CAD build for the part. Positions are in the model's coordinates, mm. Face numbers are marked on the shaded views. A direction names the side the tool comes from. Round coordinates to 2 decimals unless told otherwise and drop trailing zeros. Order: outer loops, then holes, each group sorted by start corner. A loop starts at its lowest first (then second) coordinate and runs counter-clockwise, first axis right, second up. Notation, with made-up numbers: (26.25, -34) -> (71.25, -34) arc R30 cw to (71.25, 0) -> close; hole circle Ø9 at (10, 72.5). An arc over 180 degrees is marked (long way). Answer as CSV lines item,"result". Start each with the question number.
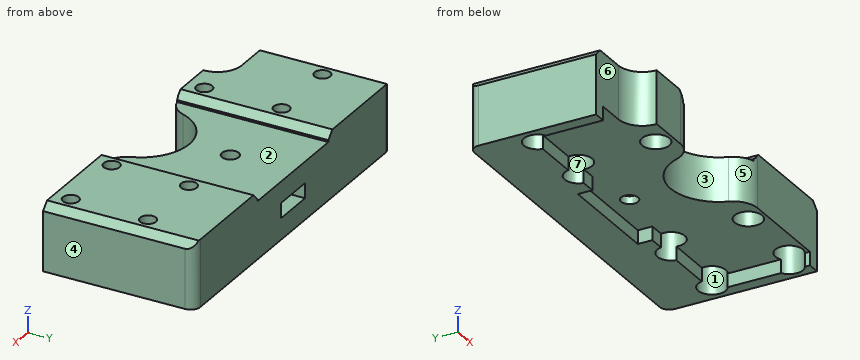
from build123d import *

# Parameters (mm, degrees)
CROQUIS1_W                  = 72
CROQUIS1_H                  = 35.8
SALIENTE_EXTRUIR1_DEPTH     = 23
CORTAR_EXTRUIR2_DEPTH       = 2.8
CROQUIS3_W                  = 5.9
CROQUIS3_H                  = 3.1
CORTAR_EXTRUIR3_DEPTH       = 7.91
SALIENTE_EXTRUIR3_DEPTH     = 3.1
CROQUIS7_W                  = 72
CROQUIS7_H                  = 22
CORTAR_EXTRUIR6_DEPTH       = 37.91
CORTAR_EXTRUIR8_DEPTH       = 15
CORTAR_EXTRUIR8_DEPTH_BACK  = 15
CROQUIS9_R                  = 1.75
CROQUIS11_R                 = 10
CORTAR_EXTRUIR10_DEPTH      = 10
REDONDEO1_R                 = 5
CROQUIS12_W                 = 72
CROQUIS12_H                 = 13.8
CROQUIS12_W_2               = 5.9
CROQUIS12_H_2               = 3.1
SALIENTE_EXTRUIR4_DEPTH     = 3.5
CROQUIS13_R                 = 1.65
CORTAR_EXTRUIR11_DEPTH      = 33.5
CORTAR_EXTRUIR12_DEPTH      = 33.5
CORTAR_EXTRUIR12_DEPTH_BACK = 3
CROQUIS14_R                 = 2.85
CROQUIS15_W                 = 26
CROQUIS15_H                 = 1.9
CORTAR_EXTRUIR13_DEPTH      = 43
CHAFL_N1_SIZE               = 1.5
CHAFL_N2_SIZE               = 1.5
CROQUIS16_W                 = 13.15
CROQUIS16_H                 = 5.14
CORTAR_EXTRUIR14_DEPTH      = 20
REDONDEO3_R                 = 5
CROQUIS17_W                 = 8.9
CROQUIS17_H                 = 3.1
SALIENTE_EXTRUIR5_DEPTH     = 4.95
REDONDEO4_R                 = 2


with BuildPart() as part:
    # Croquis1 → Saliente-Extruir1 (new body)
    with BuildSketch(Plane(origin=(0, 0, 0), x_dir=(1, 0, 0), z_dir=(0, 1, 0))):
        with Locations((36, 17.9)):
            Rectangle(CROQUIS1_W, CROQUIS1_H)
    extrude(amount=SALIENTE_EXTRUIR1_DEPTH)

    # Croquis2 → Cortar-Extruir2 (cut)
    with BuildSketch(Plane(origin=(0, 0, -35.8), x_dir=(-1, 0, 0), z_dir=(0, 0, -1))):
        Polygon((-69.4, 20), (-47, 20), (-47, 23), (-25, 23), (-25, 20), (-2.6, 20), (-2.6, -5), (-69.4, -5), align=None)
    extrude(amount=-CORTAR_EXTRUIR2_DEPTH, mode=Mode.SUBTRACT)

    # Croquis3 → Cortar-Extruir3 (cut)
    with BuildSketch(Plane(origin=(0, 23, 0), x_dir=(1, 0, 0), z_dir=(0, 1, 0))):
        with Locations((36, 29.85)):
            Rectangle(CROQUIS3_W, CROQUIS3_H)
    extrude(amount=-CORTAR_EXTRUIR3_DEPTH, mode=Mode.SUBTRACT)

    # Croquis4 → Saliente-Extruir3 (add)
    with BuildSketch(Plane(origin=(0, 0, -28.3), x_dir=(-1, 0, 0), z_dir=(0, 0, -1))):
        Polygon((-33.05, 16.793183294), (-36, 15.09), (-33.05, 15.09), align=None)
        Polygon((-36, 15.09), (-38.95, 16.793183294), (-38.95, 15.09), align=None)
    extrude(amount=SALIENTE_EXTRUIR3_DEPTH)

    # Croquis7 → Cortar-Extruir6 (cut)
    with BuildSketch(Plane(origin=(0, 23, 0), x_dir=(1, 0, 0), z_dir=(0, 1, 0))):
        with Locations((36, 11)):
            Rectangle(CROQUIS7_W, CROQUIS7_H)
    extrude(amount=-CORTAR_EXTRUIR6_DEPTH, mode=Mode.SUBTRACT)

    # Croquis9 → Cortar-Extruir8 (cut, two sides: drawn at the far end of the back side and taken through both)
    with BuildSketch(Plane(origin=(0, 0, -28.3), x_dir=(-1, 0, 0), z_dir=(0, 0, -1)).offset(-CORTAR_EXTRUIR8_DEPTH_BACK)):
        with Locations(Location((-36, 18.496366588, 0), (0, 0, 180))):
            Circle(CROQUIS9_R)
    extrude(amount=CORTAR_EXTRUIR8_DEPTH + CORTAR_EXTRUIR8_DEPTH_BACK, mode=Mode.SUBTRACT)

    # Croquis11 → Cortar-Extruir10 (cut)
    with BuildSketch(Plane(origin=(0, 0, -33), x_dir=(-1, 0, 0), z_dir=(0, 0, -1))):
        with Locations((-36, 0)):
            Circle(CROQUIS11_R)
    extrude(amount=-CORTAR_EXTRUIR10_DEPTH, mode=Mode.SUBTRACT)

    # Redondeo1
    redondeo1_edges = [part.edges().sort_by_distance(p)[0] for p in [
        (26, 0, -28),
        (46, 0, -28),
    ]]
    fillet(redondeo1_edges, radius=REDONDEO1_R)

    # Croquis12 → Saliente-Extruir4 (add)
    with BuildSketch(Plane(origin=(0, 23, 0), x_dir=(1, 0, 0), z_dir=(0, 1, 0))):
        with Locations((36, 28.9)):
            Rectangle(CROQUIS12_W, CROQUIS12_H)
        with Locations((36, 29.85)):
            Rectangle(CROQUIS12_W_2, CROQUIS12_H_2, mode=Mode.SUBTRACT)
    extrude(amount=SALIENTE_EXTRUIR4_DEPTH)

    # Croquis13 → Cortar-Extruir11 (cut)
    with BuildSketch(Plane.XY.offset(-22)):
        with Locations((19, 3.5)):
            Circle(CROQUIS13_R)
        with Locations((19, 19.5)):
            Circle(CROQUIS13_R)
        with Locations((4, 19.5)):
            Circle(CROQUIS13_R)
        with Locations((53, 3.5)):
            Circle(CROQUIS13_R)
        with Locations(Location((68, 3.5, 0), (0, 0, 31.9527464))):
            Circle(CROQUIS13_R)
        with Locations(Location((68, 19.5, 0), (0, 0, 328.0472536))):
            Circle(CROQUIS13_R)
        with Locations(Location((53, 19.5, 0), (0, 0, 17.639701394))):
            Circle(CROQUIS13_R)
    extrude(amount=-CORTAR_EXTRUIR11_DEPTH, mode=Mode.SUBTRACT)

    # Croquis14 → Cortar-Extruir12 (cut, two sides: drawn at the far end of the back side and taken through both)
    with BuildSketch(Plane(origin=(0, 0, -33), x_dir=(-1, 0, 0), z_dir=(0, 0, -1)).offset(-CORTAR_EXTRUIR12_DEPTH_BACK)):
        with Locations(Location((-53, 19.5, 0), (0, 0, 169.895817284))):
            Circle(CROQUIS14_R)
        with Locations(Location((-53, 3.5, 0), (0, 0, 180))):
            Circle(CROQUIS14_R)
        with Locations(Location((-68, 3.5, 0), (0, 0, 240.578668933))):
            Circle(CROQUIS14_R)
        with Locations(Location((-68, 19.5, 0), (0, 0, 240.578668933))):
            Circle(CROQUIS14_R)
        with Locations(Location((-19, 3.5, 0), (0, 0, 180))):
            Circle(CROQUIS14_R)
        with Locations(Location((-19, 19.5, 0), (0, 0, 169.895817284))):
            Circle(CROQUIS14_R)
        with Locations(Location((-4, 19.5, 0), (0, 0, 169.895817284))):
            Circle(CROQUIS14_R)
    extrude(amount=CORTAR_EXTRUIR12_DEPTH + CORTAR_EXTRUIR12_DEPTH_BACK, mode=Mode.SUBTRACT)

    # Croquis15 → Cortar-Extruir13 (cut)
    with BuildSketch(Plane(origin=(0, 26.5, 0), x_dir=(1, 0, 0), z_dir=(0, 1, 0))):
        with Locations((36, 22.95)):
            Rectangle(CROQUIS15_W, CROQUIS15_H)
    extrude(amount=-CORTAR_EXTRUIR13_DEPTH, mode=Mode.SUBTRACT)

    # Chaflán1
    chafl_n1_edges = [part.edges().sort_by_distance(p)[0] for p in [
        (49, 13.25, -22),
        (23, 13.25, -22),
        (72, 13.25, -22),
        (0, 13.25, -22),
    ]]
    chamfer(chafl_n1_edges, length=CHAFL_N1_SIZE)

    # Chaflán2
    chafl_n2_edges = [part.edges().sort_by_distance(p)[0] for p in [
        (33.05, 26.5, -29.85),
        (38.95, 26.5, -29.85),
    ]]
    chamfer(chafl_n2_edges, length=CHAFL_N2_SIZE)

    # Croquis16 → Cortar-Extruir14 (cut)
    with BuildSketch(Plane(origin=(0, 0, -35.8), x_dir=(-1, 0, 0), z_dir=(0, 0, -1))):
        with Locations((-6.575, 2.57)):
            Rectangle(CROQUIS16_W, CROQUIS16_H)
    extrude(amount=-CORTAR_EXTRUIR14_DEPTH, mode=Mode.SUBTRACT)

    # Redondeo3
    redondeo3_edges = [part.edges().sort_by_distance(p)[0] for p in [
        (13.15, 5.14, -27.5),
    ]]
    fillet(redondeo3_edges, radius=REDONDEO3_R)

    # Croquis17 → Saliente-Extruir5 (add)
    with BuildSketch(Plane(origin=(0, 26.5, 0), x_dir=(1, 0, 0), z_dir=(0, 1, 0))):
        Polygon((70.5, 22), (72, 23.5), (72, 35.8), (0, 35.8), (0, 23.5), (1.5, 22), (21.5, 22), (23, 23.5), (23, 23.9), (49, 23.9), (49, 23.5), (50.5, 22), align=None)
        with Locations((36, 29.85)):
            Rectangle(CROQUIS17_W, CROQUIS17_H, mode=Mode.SUBTRACT)
    extrude(amount=SALIENTE_EXTRUIR5_DEPTH)

    # Redondeo4
    redondeo4_edges = [part.edges().sort_by_distance(p)[0] for p in [
        (72, 31.45, -29.65),
        (0, 31.45, -29.65),
    ]]
    fillet(redondeo4_edges, radius=REDONDEO4_R)


solid = part.part
Item 1: Pin check, flat tips, straight feed: pin 1 (2 mm diameter, centred on x = 48.5, z = -34.5, fed in from -Y); pin 2 (1.4 mm diameter, centred on x = 34.5, z = -34.5, fed in from -Y); pin 3 (3 mm diameter, centred on x = 35.5, z = -25.5, fed in from -Y); pin 4 (2 mm diameter, centred on x = 53, y = 19.5, fed in from -Z). Stop position of each tip, or through.
Item 2: Band-saw the part on C-C, the plane y = 16. Give the cut face in (x, z).
Item 3: Band-saw the part on D-D, the plane y = 12. Give the cut face in (x, z), and give its area (3 significant figures).
Item 4: Band-saw the part on B-B, the plane x = 4. Give the cut face in (y, z).
Item 5: Tool access for the marked faces 1, 2 and 3: list every direction of +Z, -Z, +X, -X, +Y, -Y with a clear straight run to the whole face (end or side of a thin tool).
Item 6: Mould opens along X. For the marked faces 4, 5, 6 and 7 say: released by +X, released by -X, zero draft, split by the parting line, or undercut.
Item 7: Band-saw the part on A-A, the plane x = 68. Give the cut face in (y, z).
Item 8: Probe line 1 (Y direction, x = 53, z = -27.25); line 2 (X direction, y = 19.5, z = -33.05); line 3 (Y direction, x = 36, z = -32). List the from-to ranges inside material, lowest first.
Values:
1,pin 1,"y = 20"
1,pin 2,"y = 23"
1,pin 3,"y = 9.8"
1,pin 4,"through"
2,outline,"(0, -35.8) -> (2.6, -35.8) -> (2.6, -33) -> (69.4, -33) -> (69.4, -35.8) -> (72, -35.8) -> (72, -23.5) -> (70.5, -22) -> (50.5, -22) -> (49, -23.5) -> (49, -23.9) -> (23, -23.9) -> (23, -23.5) -> (21.5, -22) -> (1.5, -22) -> (0, -23.5) -> close; hole (34.42, -31.4) -> (37.58, -31.4) -> (37.58, -28.3) -> (34.42, -28.3) -> close"
3,outline,"(0, -35.8) -> (2.6, -35.8) -> (2.6, -33) -> (69.4, -33) -> (69.4, -35.8) -> (72, -35.8) -> (72, -23.5) -> (70.5, -22) -> (50.5, -22) -> (49, -23.5) -> (49, -23.9) -> (23, -23.9) -> (23, -23.5) -> (21.5, -22) -> (1.5, -22) -> (0, -23.5) -> close"
3,area,"753 mm²"
4,outline,"(5.14, -33) -> (16.65, -33) -> (16.65, -30) -> (17.85, -30) -> (17.85, -22) -> (5.14, -22) -> close; (21.15, -30) -> (22.35, -30) -> (22.35, -35.8) -> (31.45, -35.8) -> (31.45, -22) -> (21.15, -22) -> close"
5,face 1,"-Z"
5,face 2,"+Z, +Y, -Y"
5,face 3,"+Z, -Z, -Y"
6,face 4,"released by +X"
6,face 5,"undercut"
6,face 6,"zero draft"
6,face 7,"undercut"
7,outline,"(0, -33) -> (0.65, -33) -> (0.65, -30) -> (1.85, -30) -> (1.85, -22) -> (0, -22) -> close; (5.15, -30) -> (6.35, -30) -> (6.35, -33) -> (16.65, -33) -> (16.65, -30) -> (17.85, -30) -> (17.85, -22) -> (5.15, -22) -> close; (21.15, -30) -> (22.35, -30) -> (22.35, -35.8) -> (31.45, -35.8) -> (31.45, -22) -> (21.15, -22) -> close"
8,line 1,"0 to 1.85, 5.15 to 17.85, 21.15 to 31.45"
8,line 2,"0 to 1.15, 70.85 to 72"
8,line 3,"10 to 16.75, 20.25 to 31.45"
